from build123d import *

# Parameters (mm, degrees)
F0_W     = 5
F0_H     = 5
F1_DEPTH = 5
F2_D     = 3
F3_R     = 2.49999
F4_W     = 4
F4_H     = 5
F5_DEPTH = 9.5


# Not quite as in the source:
# - a fillet or chamfer is up to 0.001 mm smaller than in the source, because OpenCascade refuses the exact size


with BuildPart() as f1:
    # F0 (on Front) → F1 (new body)
    with BuildSketch(Plane.XZ):
        Polygon((4.8, 5), (9.8, 5), (9.8, 15), (9.8, 20), (4.8, 20), align=None)
        with Locations((7.3, 22.5)):
            Rectangle(F0_W, F0_H)
    extrude(amount=F1_DEPTH)

    # F2 (through all)
    with Locations(Plane(origin=(0, 0, 0), x_dir=(1, 0, 0), z_dir=(0, 1, 0))):
        with Locations((7.3, -22.5)):
            Hole(F2_D / 2)

    # F3 (radius 2.5 in the source; OpenCascade refuses exactly that, so slightly less here)
    f3_edges = [f1.edges().sort_by_distance(p)[0] for p in [
        (4.8, -2.5, 25),
        (9.8, -2.5, 25),
    ]]
    fillet(f3_edges, radius=F3_R)

    # F4 (on face) → F5 (join)
    with BuildSketch(Plane.YZ.offset(9.8)):
        with Locations((-2.5, 2.5)):
            Rectangle(F4_W, F4_H)
    extrude(amount=-F5_DEPTH)


solid = f1.part
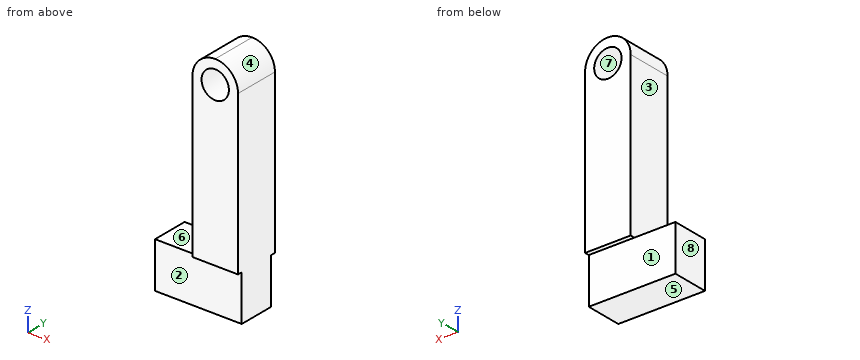
Model file for the job. Use its own axes, mm. Face numbers are marked on the shaded views. A direction names the side the tool comes from. Round coordinates to 2 decimals unless told otherwise and drop trailing zeros. Loops run counter-clockwise (first coordinate to the right, second up) from the corner with the lowest first, then second, coordinate; pieces in that order, holes last.
1. Band-saw the part on C-C, the plane z = 9.5. List the corners of the cut face in (x, y).
Check values:
outline: (4.8, -5) - (9.8, -5) - (9.8, 0) - (4.8, 0) - close
2. Tool access for the marked faces 1, 2, 3, 4 and 5: list every direction of +Z, -Z, +X, -X, +Y, -Y with a clear straight run to the whole face (end or side of a thin tool).
Check values:
face 1: -Z, +X, -X, +Y
face 2: -Z, +X, -X, -Y
face 3: +Z, -X, +Y, -Y
face 4: +Z, +X, +Y, -Y
face 5: -Z, +X, -X, +Y, -Y
3. Wall check: probe 1 along Z at (x, y) = (7.3, -2.65); probe 2 along X at (y, z) = (-4.45, 22.5); probe 3 along X at (y, z) = (-0.8, 17.5). Give the ranges that are in metal, low to high.
Check values:
probe 1: z = 0 to 21, 24 to 25
probe 2: x = 4.8 to 5.8, 8.8 to 9.8
probe 3: x = 4.8 to 9.8
4. Band-saw the part on B-B, the plane x = 7. List the corners of the cut face in (y, z), and give its area (3 significant figures).
Check values:
outline: (-5, 5) - (-4.5, 5) - (-4.5, 0) - (-0.5, 0) - (-0.5, 5) - (0, 5) - (0, 21.03) - (-5, 21.03) - close; (-5, 23.97) - (0, 23.97) - (0, 24.98) - (-5, 24.98) - close
area: 105 mm2
5. Mould opens along Z. For the marked faces 6, 7 and 8 say: +Z half, -Z half, draft (parallel to the pull), parting line (faces both ways), or undercut.
Check values:
face 6: +Z half
face 7: undercut
face 8: draft
6. Band-saw the part on D-D, the plane x = 3.5. List the corners of the cut face in (y, z), and give its area (3 significant figures).
Check values:
outline: (-4.5, 0) - (-0.5, 0) - (-0.5, 5) - (-4.5, 5) - close
area: 20.0 mm2
7. Drop flat-ended pins along their axis: P1, Ø1, axis at x = 6.5, y = -3.5, coming from the +Z side; P2, Ø2.5, axis at y = -2.5, z = 15, coming from the -X side; P3, Ø1.5, axis at x = 5, z = 1.5, coming from the +Y side. Give the stop position or say it passes through.
Check values:
P1: stops at z = 24.98
P2: stops at x = 4.8
P3: stops at y = -0.5
